Check sheet for the modelled part. Datum: model origin and axes. Units: mm. A direction names the side the tool comes from. Coordinates: 2 decimals unless noted, no trailing zeros. Write each loop counter-clockwise with the first axis right and the second up, starting at its lowest first coordinate (ties: lowest second). Pieces come first, ordered by that corner, then holes. Notation, with made-up numbers: M -4,53.25 L 15,53.25 A21 cw 15,75.25 Z; hole C 38,2 d1. An arc over 180 degrees is marked long. Answer as CSV lines item,"result".
from build123d import *

# Parameters (mm, degrees)
F0_W           = 50
F0_H           = 25
F1_DEPTH       = 10
F2_D           = 5.5
F2_DEPTH       = 14
F2_CBORE_D     = 9.75
F2_CBORE_DEPTH = 5
F2_TIP         = 1.6523667023


with BuildPart() as f1:
    # F0 (on Front) → F1 (new body)
    with BuildSketch(Plane.XZ):
        Rectangle(F0_W, F0_H)
    extrude(amount=-F1_DEPTH)

    # F2
    with Locations(Plane.XZ):
        with Locations((-12, 6.5), (12, 6.5), (12, -6.5)):
            CounterBoreHole(F2_D / 2, F2_CBORE_D / 2, F2_CBORE_DEPTH, depth=F2_DEPTH)
            with Locations((0, 0, -(F2_DEPTH + F2_TIP / 2))):  # 118° drill point
                Cone(0, F2_D / 2, F2_TIP, mode=Mode.SUBTRACT)


solid = f1.part
1) Section check C-C, the plane y = 9.25. Record the boundary of the cut face in (x, z).
Answer key:
outline,"M -25,-12.5 L 25,-12.5 L 25,12.5 L -25,12.5 Z; hole C -12,6.5 d5.5; hole C 12,-6.5 d5.5; hole C 12,6.5 d5.5"
2) Mould release check, pull along Z, two halves, no side actions. Record for faces 1 (the face through (0, 5, 12.5)), 2 (the face through (0, 0, 0)), 3 (the face through (8.407, 2.465, -3.205)), 4 (the face through (-13.06, 2.46, 1.74)): pulls with the +Z half, pulls with the -Z half, needs draft (parallel to the pull), parting line crosses it, or undercut.
Answer key:
face 1,"pulls with the +Z half"
face 2,"needs draft"
face 3,"undercut"
face 4,"undercut"
3) Tool access check on faces 5 (the face through (9.46, 7.54, -7.55)), 6 (the face through (-10, 5, 4)). Record the directions out of +Z, -Z, +X, -X, +Y, -Y that give a thin tool (end or side, any length) a straight path to the whole face; none if there is none.
Answer key:
face 5,"+Y, -Y"
face 6,"-Y"
4) Thickness scan on line 1 along Z through (x, y) = (12, 1.3) (3 decimals); line 2 along Z through (x, y) = (12.5, 5.5); line 3 along X through (y, z) = (3, 9). Record the ranges inside material, lowest first.
Answer key:
line 1,"z = -12.5 to -11.375, -1.625 to 1.625, 11.375 to 12.5"
line 2,"z = -12.5 to -9.2, -3.8 to 3.8, 9.2 to 12.5"
line 3,"x = -25 to -16.19, -7.81 to 7.81, 16.19 to 25"
5) Section check D-D, the plane z = 6.5. Record the boundary of the cut face in (x, y) (3 decimals), plus the area to 4 significant figures.
Answer key:
outline,"M -25,0 L -16.875,0 L -16.875,5 L -14.75,5 L -14.75,10 L -25,10 Z; M -9.25,5 L -7.125,5 L -7.125,0 L 7.125,0 L 7.125,5 L 9.25,5 L 9.25,10 L -9.25,10 Z; M 14.75,5 L 16.875,5 L 16.875,0 L 25,0 L 25,10 L 14.75,10 Z"
area,"347.5 mm2"
6) Section check A-A, the plane z = -6.5. Record the boundary of the cut face in (x, y) (3 decimals).
Answer key:
outline,"M -25,0 L 7.125,0 L 7.125,5 L 9.25,5 L 9.25,10 L -25,10 Z; M 14.75,5 L 16.875,5 L 16.875,0 L 25,0 L 25,10 L 14.75,10 Z"
7) Section check B-B, the plane x = 12. Record the boundary of the cut face in (y, z) (3 decimals).
Answer key:
outline,"M 0,-12.5 L 10,-12.5 L 10,-9.25 L 5,-9.25 L 5,-11.375 L 0,-11.375 Z; M 0,-1.625 L 5,-1.625 L 5,-3.75 L 10,-3.75 L 10,3.75 L 5,3.75 L 5,1.625 L 0,1.625 Z; M 0,11.375 L 5,11.375 L 5,9.25 L 10,9.25 L 10,12.5 L 0,12.5 Z"
8) Depth check by flat-ended pin: P1, Ø8, axis at x = 12, z = -6.5, coming from the -Y side; P2, Ø4.5, axis at x = 12, z = 6.5, coming from the -Y side. Enter the tip coordinate at first touch or a pass-through.
Answer key:
P1,"stops at y = 5"
P2,"passes through"
